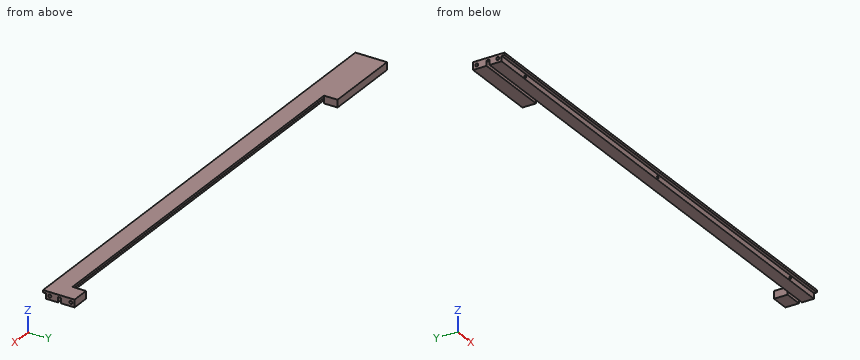
```python
from build123d import *

# Parameters (mm, degrees)
BOSS_EXTRUDE1_DEPTH = 10
SKETCH2_W           = 657
SKETCH2_H           = 4
CUT_EXTRUDE1_DEPTH  = 7
SKETCH3_W           = 657
SKETCH3_H           = 4
CUT_EXTRUDE2_DEPTH  = 7
SKETCH4_R           = 1.5
CUT_EXTRUDE3_DEPTH  = 12
SKETCH6_R           = 2
CUT_EXTRUDE4_DEPTH  = 10
CUT_EXTRUDE5_START  = -10
SKETCH7_R           = 2
CUT_EXTRUDE5_DEPTH  = 10


with BuildPart() as part:
    # Sketch1 → Boss-Extrude1 (new body)
    with BuildSketch(Plane.XY):
        Polygon((-482.706212002, 28.610388863), (-482.706212002, -13.389611137), (174.293787998, -13.389611137), (174.293787998, 28.610388863), (150.293787998, 28.610388863), (150.293787998, 10.610388863), (-378.706212002, 10.610388863), (-378.706212002, 28.610388863), align=None)
    extrude(amount=BOSS_EXTRUDE1_DEPTH)

    # Sketch2 → Cut-Extrude1 (cut)
    with BuildSketch(Plane(origin=(0, 0, 0), x_dir=(-1, 0, 0), z_dir=(0, 0, -1))):
        with Locations((154.206212002, 8.610388863)):
            Rectangle(SKETCH2_W, SKETCH2_H)
    extrude(amount=-CUT_EXTRUDE1_DEPTH, mode=Mode.SUBTRACT)

    # Sketch3 → Cut-Extrude2 (cut)
    with BuildSketch(Plane(origin=(0, 0, 0), x_dir=(-1, 0, 0), z_dir=(0, 0, -1))):
        with Locations((154.206212002, -11.389611137)):
            Rectangle(SKETCH3_W, SKETCH3_H)
    extrude(amount=-CUT_EXTRUDE2_DEPTH, mode=Mode.SUBTRACT)

    # Sketch4 → Cut-Extrude3 (cut)
    with BuildSketch(Plane.XZ.offset(9.389611137)):
        with Locations(Location((-432.706212002, 3.5, 0), (0, 0, 270))):
            Circle(SKETCH4_R)
        with Locations(Location((-154.206212002, 3.5, 0), (0, 0, 270))):
            Circle(SKETCH4_R)
        with Locations(Location((124.293787998, 3.5, 0), (0, 0, 270))):
            Circle(SKETCH4_R)
    extrude(amount=-CUT_EXTRUDE3_DEPTH, mode=Mode.SUBTRACT)

    # Sketch6 → Cut-Extrude4 (cut)
    with BuildSketch(Plane(origin=(174.293787998, 0, 0), x_dir=(0, 0, -1), z_dir=(1, 0, 0))):
        with Locations((-5, 23.610388863)):
            Circle(SKETCH6_R)
        with Locations((-5, -4.389611137)):
            Circle(SKETCH6_R)
    extrude(amount=-CUT_EXTRUDE4_DEPTH, mode=Mode.SUBTRACT)

    # Sketch7 → Cut-Extrude5 (cut)
    with BuildSketch(Plane.ZY.offset(482.706212002).offset(CUT_EXTRUDE5_START)):
        with Locations(Location((5, 23.610388863, 0), (0, 0, 180))):
            Circle(SKETCH7_R)
        with Locations(Location((5, -4.389611137, 0), (0, 0, 180))):
            Circle(SKETCH7_R)
    extrude(amount=CUT_EXTRUDE5_DEPTH, mode=Mode.SUBTRACT)


solid = part.part
```
Geometry check sheet. Reference: the model listing, model coordinates, mm. Round coordinates to 2 decimals unless told otherwise and drop trailing zeros. Loops run counter-clockwise (first coordinate to the right, second up) from the corner with the lowest first, then second, coordinate; pieces in that order, holes last. Notation, with made-up numbers: (-23.5, 18.5) - (7.5, 18.5) arc R12 ccw to (7.5, 38.5) - close; hole circle Ø3 at (-31, -26.5). An arc over 180 degrees is marked (long way). Write each question's results on one line, items separated by ' | '. Start each with the question number.
Q1. Cross-section at B-B on z = 8.5. Enter the section's corners in (x, y), and give its area (3 significant figures).
Q2. Cross-section at C-C on x = 135. Enter the section's corners in (y, z), and give its area (3 significant figures).
Q3. Gauge pin test, flat ends, axial feed: P1, Ø3.5, axis at x = -16.5, z = 4, coming from the +Y side; P2, Ø3, axis at y = -4, z = 4.5, coming from the -X side; P3, Ø3.5, axis at x = -146.5, z = 8, coming from the +Y side; P4, Ø1.2, axis at y = -5, z = 5.5, coming from the +X side. Record the tip position at first contact, or that the pin passes through.
Q4. Thickness scan on line 1 (Y direction, x = 172, z = 5); line 2 (X direction, y = -6, z = 3.5); line 3 (X direction, y = 25, z = 3.75). Record the ranges inside material, lowest first. Write a range as [from, to].
Q5. Cross-section at A-A on x = -407. Enter the section's corners in (y, z).
Answers below:
1) outline: (-482.71, -13.39) - (174.29, -13.39) - (174.29, 28.61) - (150.29, 28.61) - (150.29, 10.61) - (-378.71, 10.61) - (-378.71, 28.61) - (-482.71, 28.61) - close | area: 18,100 mm²
2) outline: (-13.39, 7) - (-9.39, 7) - (-9.39, 0) - (6.61, 0) - (6.61, 7) - (10.61, 7) - (10.61, 10) - (-13.39, 10) - close | area: 184 mm²
3) P1: stops at y = 6.61 | P2: stops at x = -482.71 | P3: stops at y = 10.61 | P4: stops at x = 164.29
4) line 1: y = [-9.39, -6.39], [-2.39, 6.61], [10.61, 21.61], [25.61, 28.61] | line 2: x = [-482.71, -434.21], [-431.21, -155.71], [-152.71, 122.79], [125.79, 174.29] | line 3: x = [-472.71, -378.71], [150.29, 164.29]
5) outline: (-13.39, 7) - (-9.39, 7) - (-9.39, 0) - (6.61, 0) - (6.61, 7) - (10.61, 7) - (10.61, 0) - (28.61, 0) - (28.61, 10) - (-13.39, 10) - close
